Design review of the part built by this model. Coordinates are the model's own, in mm. Face numbers are marked on the shaded views. A direction names the side the tool comes from. Give positions to 0.01 mm unless a question says otherwise; leave off trailing zeros. Order: outer loops, then holes, each group sorted by start corner. A loop starts at its lowest first (then second) coordinate and runs counter-clockwise, first axis right, second up. Notation, with made-up numbers: M 24,-15 L 45,-15 A19 ccw 45,4 Z; hole C 48,-30 d11. An arc over 180 degrees is marked long. Answer as a JSON object with one key per item and string values.
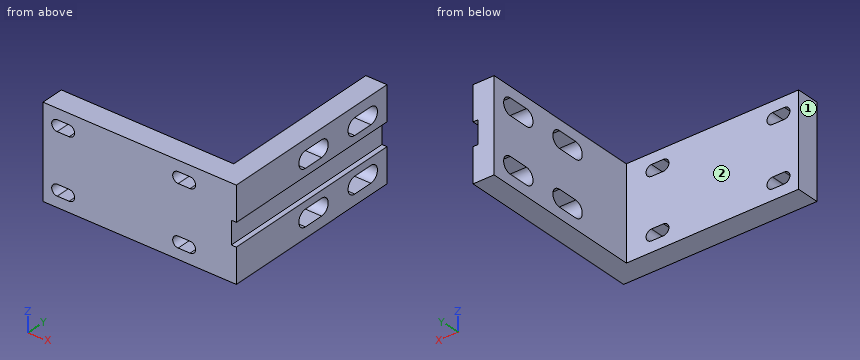
from build123d import *

# Parameters (mm, degrees)
SKETCH_1_W          = 23
SKETCH_1_H          = 205
EXTRUDE_1_DEPTH     = 100
SKETCH_3_W          = 188
SKETCH_3_H          = 25
EXTRUDE_3_DEPTH     = 100
CUT_EXTRUDE_1_REACH = 312.719
CUT_EXTRUDE_2_REACH = 312.719
SKETCH_6_W          = 25
SKETCH_6_H          = 205
CUT_EXTRUDE_3_DEPTH = 5.5


with BuildPart() as part:
    # 草图1 → 凸台-拉伸1 (new body)
    with BuildSketch(Plane.XY):
        with Locations((-11.5, -102.5)):
            Rectangle(SKETCH_1_W, SKETCH_1_H)
    extrude(amount=EXTRUDE_1_DEPTH)

    # 草图3 → 凸台-拉伸3 (add)
    with BuildSketch(Plane.XY.offset(100)):
        with Locations((-117, -192.5)):
            Rectangle(SKETCH_3_W, SKETCH_3_H)
    extrude(amount=-EXTRUDE_3_DEPTH)

    # 草图4 → 切除-拉伸1 (cut, up to next)
    with BuildSketch(Plane(origin=(0, 0, 0), x_dir=(0, 0, -1), z_dir=(1, 0, 0)), mode=Mode.PRIVATE) as cut_extrude_1_sk1:
        with BuildLine():
            Line((-70.5, -22), (-70.5, -44))
            ThreePointArc((-70.5, -44), (-79.5, -53), (-88.5, -44))
            Line((-88.5, -44), (-88.5, -22))
            ThreePointArc((-88.5, -22), (-79.5, -13), (-70.5, -22))
        make_face()
    cut_extrude_1_tool1 = extrude(cut_extrude_1_sk1.sketch, amount=-CUT_EXTRUDE_1_REACH, mode=Mode.PRIVATE) & part.part
    # 草图4 → 切除-拉伸1 (cut, up to next)
    with BuildSketch(Plane(origin=(0, 0, 0), x_dir=(0, 0, -1), z_dir=(1, 0, 0)), mode=Mode.PRIVATE) as cut_extrude_1_sk2:
        with BuildLine():
            Line((-11.5, -22), (-11.5, -44))
            ThreePointArc((-11.5, -44), (-20.5, -53), (-29.5, -44))
            Line((-29.5, -44), (-29.5, -22))
            ThreePointArc((-29.5, -22), (-20.5, -13), (-11.5, -22))
        make_face()
    cut_extrude_1_tool2 = extrude(cut_extrude_1_sk2.sketch, amount=-CUT_EXTRUDE_1_REACH, mode=Mode.PRIVATE) & part.part
    # 草图4 → 切除-拉伸1 (cut, up to next)
    with BuildSketch(Plane(origin=(0, 0, 0), x_dir=(0, 0, -1), z_dir=(1, 0, 0)), mode=Mode.PRIVATE) as cut_extrude_1_sk3:
        with BuildLine():
            Line((-70.5, -89), (-70.5, -111))
            ThreePointArc((-70.5, -111), (-79.5, -120), (-88.5, -111))
            Line((-88.5, -111), (-88.5, -89))
            ThreePointArc((-88.5, -89), (-79.5, -80), (-70.5, -89))
        make_face()
    cut_extrude_1_tool3 = extrude(cut_extrude_1_sk3.sketch, amount=-CUT_EXTRUDE_1_REACH, mode=Mode.PRIVATE) & part.part
    # 草图4 → 切除-拉伸1 (cut, up to next)
    with BuildSketch(Plane(origin=(0, 0, 0), x_dir=(0, 0, -1), z_dir=(1, 0, 0)), mode=Mode.PRIVATE) as cut_extrude_1_sk4:
        with BuildLine():
            Line((-11.5, -89), (-11.5, -111))
            ThreePointArc((-11.5, -111), (-20.5, -120), (-29.5, -111))
            Line((-29.5, -111), (-29.5, -89))
            ThreePointArc((-29.5, -89), (-20.5, -80), (-11.5, -89))
        make_face()
    cut_extrude_1_tool4 = extrude(cut_extrude_1_sk4.sketch, amount=-CUT_EXTRUDE_1_REACH, mode=Mode.PRIVATE) & part.part
    add(cut_extrude_1_tool1.solids().sort_by_distance((0, -33, 79.5))[0], mode=Mode.SUBTRACT)
    add(cut_extrude_1_tool2.solids().sort_by_distance((0, -33, 20.5))[0], mode=Mode.SUBTRACT)
    add(cut_extrude_1_tool3.solids().sort_by_distance((0, -100, 79.5))[0], mode=Mode.SUBTRACT)
    add(cut_extrude_1_tool4.solids().sort_by_distance((0, -100, 20.5))[0], mode=Mode.SUBTRACT)

    # 草图5 → 切除-拉伸2 (cut, up to next)
    with BuildSketch(Plane.XZ.offset(205), mode=Mode.PRIVATE) as cut_extrude_2_sk1:
        with BuildLine():
            Line((-195.5, 88.5), (-182.5, 88.5))
            ThreePointArc((-182.5, 88.5), (-176.5, 82.5), (-182.5, 76.5))
            Line((-182.5, 76.5), (-195.5, 76.5))
            ThreePointArc((-195.5, 76.5), (-201.5, 82.5), (-195.5, 88.5))
        make_face()
    cut_extrude_2_tool1 = extrude(cut_extrude_2_sk1.sketch, amount=-CUT_EXTRUDE_2_REACH, mode=Mode.PRIVATE) & part.part
    # 草图5 → 切除-拉伸2 (cut, up to next)
    with BuildSketch(Plane.XZ.offset(205), mode=Mode.PRIVATE) as cut_extrude_2_sk2:
        with BuildLine():
            Line((-63.5, 88.5), (-50.5, 88.5))
            ThreePointArc((-50.5, 88.5), (-44.5, 82.5), (-50.5, 76.5))
            Line((-50.5, 76.5), (-63.5, 76.5))
            ThreePointArc((-63.5, 76.5), (-69.5, 82.5), (-63.5, 88.5))
        make_face()
    cut_extrude_2_tool2 = extrude(cut_extrude_2_sk2.sketch, amount=-CUT_EXTRUDE_2_REACH, mode=Mode.PRIVATE) & part.part
    # 草图5 → 切除-拉伸2 (cut, up to next)
    with BuildSketch(Plane.XZ.offset(205), mode=Mode.PRIVATE) as cut_extrude_2_sk3:
        with BuildLine():
            Line((-195.5, 23.5), (-182.5, 23.5))
            ThreePointArc((-182.5, 23.5), (-176.5, 17.5), (-182.5, 11.5))
            Line((-182.5, 11.5), (-195.5, 11.5))
            ThreePointArc((-195.5, 11.5), (-201.5, 17.5), (-195.5, 23.5))
        make_face()
    cut_extrude_2_tool3 = extrude(cut_extrude_2_sk3.sketch, amount=-CUT_EXTRUDE_2_REACH, mode=Mode.PRIVATE) & part.part
    # 草图5 → 切除-拉伸2 (cut, up to next)
    with BuildSketch(Plane.XZ.offset(205), mode=Mode.PRIVATE) as cut_extrude_2_sk4:
        with BuildLine():
            Line((-63.5, 23.5), (-50.5, 23.5))
            ThreePointArc((-50.5, 23.5), (-44.5, 17.5), (-50.5, 11.5))
            Line((-50.5, 11.5), (-63.5, 11.5))
            ThreePointArc((-63.5, 11.5), (-69.5, 17.5), (-63.5, 23.5))
        make_face()
    cut_extrude_2_tool4 = extrude(cut_extrude_2_sk4.sketch, amount=-CUT_EXTRUDE_2_REACH, mode=Mode.PRIVATE) & part.part
    add(cut_extrude_2_tool1.solids().sort_by_distance((-189, -205, 82.5))[0], mode=Mode.SUBTRACT)
    add(cut_extrude_2_tool2.solids().sort_by_distance((-57, -205, 82.5))[0], mode=Mode.SUBTRACT)
    add(cut_extrude_2_tool3.solids().sort_by_distance((-189, -205, 17.5))[0], mode=Mode.SUBTRACT)
    add(cut_extrude_2_tool4.solids().sort_by_distance((-57, -205, 17.5))[0], mode=Mode.SUBTRACT)

    # 草图6 → 切除-拉伸3 (cut)
    with BuildSketch(Plane(origin=(0, 0, 0), x_dir=(0, 0, -1), z_dir=(1, 0, 0))):
        with Locations((-50, -102.5)):
            Rectangle(SKETCH_6_W, SKETCH_6_H)
    extrude(amount=-CUT_EXTRUDE_3_DEPTH, mode=Mode.SUBTRACT)


solid = part.part
(1) To check wall thickness, follow L1, parallel to Y at x = -20, z = 15; L2, parallel to Y at x = -70.5, z = 95.5; L3, parallel to X at y = -105, z = 61.5. State the ranges of each line that lie inside material, in increasing order. Write a range as from..to.
Checked values:
{"L1": "y = -205..-118.12, -81.88..-51.12, -14.88..0", "L2": "y = -205..-180", "L3": "x = -23..-5.5"}
(2) We need section A-A (x = -185). Write out the cut boundary in (y, z), plus the area to 3 significant figures.
Checked values:
{"outline": "M -205,0 L -180,0 L -180,11.5 L -205,11.5 Z; M -205,23.5 L -180,23.5 L -180,76.5 L -205,76.5 Z; M -205,88.5 L -180,88.5 L -180,100 L -205,100 Z", "area": "1,900 mm^2"}
(3) We need section C-C (z = 20.5). Write out the cut boundary in (x, y).
Checked values:
{"outline": "M -211,-205 L -200.7,-205 L -200.7,-180 L -211,-180 Z; M -177.3,-205 L -68.7,-205 L -68.7,-180 L -177.3,-180 Z; M -45.3,-205 L 0,-205 L 0,-120 L -23,-120 L -23,-180 L -45.3,-180 Z; M -23,-80 L 0,-80 L 0,-53 L -23,-53 Z; M -23,-13 L 0,-13 L 0,0 L -23,0 Z"}
(4) We need section D-D (z = 44). Write out the cut boundary in (x, y), plus the area to 3 significant figures.
Checked values:
{"outline": "M -211,-205 L -5.5,-205 L -5.5,0 L -23,0 L -23,-180 L -211,-180 Z", "area": "8,290 mm^2"}
(5) Insertion check: pin 1 (5 mm diameter, centred on y = -169.5, z = 90, fed in from -X); pin 2 (8 mm diameter, centred on y = -40.5, z = 77.5, fed in from +X); pin 3 (4 mm diameter, centred on x = -164.5, z = 44.5, fed in from +Y). Each pin has a flat end and moves straight along its axis. Give the tip position at first contact, or say it passes through.
Checked values:
{"pin 1": "stops at x = -23", "pin 2": "passes through", "pin 3": "stops at y = -180"}
(6) We need section B-B (y = -107). Write out the cut boundary in (x, z).
Checked values:
{"outline": "M -23,0 L 0,0 L 0,11.5 L -23,11.5 Z; M -23,29.5 L 0,29.5 L 0,37.5 L -5.5,37.5 L -5.5,62.5 L 0,62.5 L 0,70.5 L -23,70.5 Z; M -23,88.5 L 0,88.5 L 0,100 L -23,100 Z"}
(7) Tool access review of the marked faces 1 and 2: name each direction out of +Z, -Z, +X, -X, +Y, -Y from which nothing blocks a thin tool from reaching the whole face with its end or side.
Checked values:
{"face 1": "+Z, -Z, -X, +Y, -Y", "face 2": "+Z, -Z, -X, +Y"}
